from build123d import *

# Parameters (mm, degrees)
BOSS_EXTRUDE1_DEPTH = 17


with BuildPart() as part:
    # Sketch1 → Boss-Extrude1 (new, symmetric)
    with BuildSketch(Plane(origin=(0, 0, 0), x_dir=(1, 0, 0), z_dir=(0, 1, 0))):
        Polygon((-12, 18), (-8.25, 18), (-8.25, 15), (-14.5, 15), (-14.5, -15), (-8.25, -15), (-8.25, -12), (-12, -12), (-12, -10), (12, -10), (12, -12), (8.25, -12), (8.25, -15), (14.5, -15), (14.5, 15), (8.25, 15), (8.25, 18), (12, 18), (12, 20), (-12, 20), align=None)
    extrude(amount=BOSS_EXTRUDE1_DEPTH, both=True)


solid = part.part
CAD build for the part. Positions are in the model's coordinates, mm. A direction names the side the tool comes from. Round coordinates to 2 decimals unless told otherwise and drop trailing zeros. Loops run counter-clockwise (first coordinate to the right, second up) from the corner with the lowest first, then second, coordinate; pieces in that order, holes last. Notation, with made-up numbers: M 66.25,-18 L 75.25,-18 A8 ccw 75.25,-11 Z; hole C 50,-26.75 d4. An arc over 180 degrees is marked long. One line per question, with ' | ' between items. Start each with the question number.
Item 1: Pin check, flat tips, straight feed: pin 1 Ø1.6 at (y, z) = (-0.5, -18.5) entering from -X; pin 2 Ø1.5 at (x, y) = (-3.5, 11) entering from +Z; pin 3 Ø3.5 at (y, z) = (3, -17) entering from +X; pin 4 Ø12 at (x, y) = (3.5, 5.5) entering from +Z. Stop position of each tip, or through.
Item 2: Cut at D-D, the plane z = -16. Write the cut outline in (x, y), plus the area to 3 significant figures.
Item 3: Cut at C-C, the plane x = -7. Write the cut outline in (y, z), plus the area to 3 significant figures.
Item 4: Cut at B-B, the plane y = -4. Write the cut outline in (x, z).
Item 5: Two-plate mould, pull along Z, no slides. Class faces 1 (the flat face through (11, 0, 15)), 2 (the flat face through (-12, 0, 11)), 3 (the flat face through (10, 0, 12)), 4 (the flat face through (0, -17, -3)): pulls with the +Z half, pulls with the -Z half, needs draft (parallel to the pull), parting line crosses it, or undercut.
Item 6: Which spindle directions (+Z, -Z, +X, -X, +Y, -Y) get a long thin tool onto all of the face, cutting with end or side? Do faces 5 (the flat face through (10, 0, -18)), 6 (the flat face through (12, 0, -19)), 7 (the flat face through (-10, 0, -18)), 8 (the flat face through (12, 0, 11)). Say none if no direction does.
Item 7: Wall check: line 1 (Z direction, x = 11.25, y = -8); line 2 (X direction, y = 8.5, z = 13); line 3 (Z direction, x = 2, y = -0.5). Give the ranges that are in metal, low to high.
Item 8: Cut at A-A, the plane x = 9. Write the cut outline in (y, z).
Responses:
1) pin 1: stops at x = -12 | pin 2: stops at z = 10 | pin 3: stops at x = 12 | pin 4: stops at z = 15
2) outline: M -8.25,-17 L 8.25,-17 L 8.25,17 L -8.25,17 Z | area: 561 mm²
3) outline: M -17,-20 L 17,-20 L 17,10 L -17,10 Z | area: 1,020 mm²
4) outline: M -14.5,-15 L -8.25,-15 L -8.25,-18 L -12,-18 L -12,-20 L 12,-20 L 12,-18 L 8.25,-18 L 8.25,-15 L 14.5,-15 L 14.5,15 L 8.25,15 L 8.25,12 L 12,12 L 12,10 L -12,10 L -12,12 L -8.25,12 L -8.25,15 L -14.5,15 Z
5) face 1: pulls with the +Z half | face 2: undercut | face 3: undercut | face 4: needs draft
6) face 5: +X, +Y, -Y | face 6: -Z, +X, +Y, -Y | face 7: -X, +Y, -Y | face 8: +Y, -Y
7) line 1: z = -20 to -18, -15 to 10, 12 to 15 | line 2: x = -14.5 to -8.25, 8.25 to 14.5 | line 3: z = -20 to 10
8) outline: M -17,-20 L 17,-20 L 17,-18 L -17,-18 Z; M -17,-15 L 17,-15 L 17,10 L -17,10 Z; M -17,12 L 17,12 L 17,15 L -17,15 Z
